Autodesk Inventor part; units mm, degrees
ref_plane "YZ Plane" through (0, 0, 0) normal (1, 0, 0) x (0, 1, 0)
ref_plane "XZ Plane" through (0, 0, 0) normal (0, 1, 0) x (-1, 0, 0)
ref_plane "XY Plane" through (0, 0, 0) normal (0, 0, 1) x (1, 0, 0)
sketch "Skizze2" plane through (0, 0, 0) normal (0, 1, 0) x (-1, 0, 0)
  line L0 (0, 0) -> (30, 0)
  line L1 (30, 0) -> (30, 30)
  line L2 (30, 30) -> (0, 30)
  line L3 (0, 30) -> (0, 0)
  line L4 (28, 28) -> (2, 28)
  line L5 (2, 28) -> (2, 2)
  line L6 (2, 2) -> (28, 2)
  line L7 (28, 2) -> (28, 28)
  line L8 (19, 30) -> (19, 28)
  line L9 (11, 30) -> (11, 28)
  line L10 (23.5, 28) -> (23.5, 25)
  line L11 (19.5, 21) -> (10.5, 21)
  line L12 (6.5, 25) -> (6.5, 28)
  line L13 (23.5, 25) -> (19.5, 21)
  line L14 (6.5, 25) -> (10.5, 21)
  line L15 (5, 6.5) -> (2, 6.5)
  line L16 (9, 19.5) -> (9, 10.5)
  line L17 (5, 23.5) -> (9, 19.5)
  line L18 (2, 23.5) -> (5, 23.5)
  line L19 (0, 19) -> (2, 19)
  line L20 (0, 11) -> (2, 11)
  line L21 (5, 6.5) -> (9, 10.5)
  line L22 (23.5, 5) -> (23.5, 2)
  line L23 (10.5, 9) -> (19.5, 9)
  line L24 (6.5, 5) -> (10.5, 9)
  line L25 (6.5, 2) -> (6.5, 5)
  line L26 (11, 0) -> (11, 2)
  line L27 (19, 0) -> (19, 2)
  line L28 (23.5, 5) -> (19.5, 9)
  line L29 (25, 23.5) -> (28, 23.5)
  line L30 (21, 10.5) -> (21, 19.5)
  line L31 (25, 6.5) -> (21, 10.5)
  line L32 (28, 6.5) -> (25, 6.5)
  line L33 (30, 11) -> (28, 11)
  line L34 (30, 19) -> (28, 19)
  line L35 (25, 23.5) -> (21, 19.5)
  circle A0 centre (15, 15) radius 3.5
  line L36 (20, 30) -> (20, 29)
  line L37 (20, 29) -> (19, 29)
  line L38 (11, 29) -> (10, 29)
  line L39 (10, 29) -> (10, 30)
  line L40 (1, 10) -> (0, 10)
  line L41 (1, 11) -> (1, 10)
  line L42 (1, 20) -> (1, 19)
  line L43 (0, 20) -> (1, 20)
  line L44 (20, 1) -> (20, 0)
  line L45 (19, 1) -> (20, 1)
  line L46 (10, 1) -> (11, 1)
  line L47 (10, 0) -> (10, 1)
  line L48 (29, 20) -> (30, 20)
  line L49 (29, 19) -> (29, 20)
  line L50 (29, 10) -> (29, 11)
  line L51 (30, 10) -> (29, 10)
  point P0 (23.5, 21)
  point P1 (6.5, 21)
  point P2 (9, 6.5)
  point P3 (9, 23.5)
  point P4 (23.5, 9)
  point P5 (6.5, 9)
  point P6 (21, 23.5)
  point P7 (21, 6.5)
  dimension "d23" = 30
  dimension "d24" = 30
  dimension "d25" = 2
  dimension "d26" = 2
  dimension "d27" = 2
  dimension "d28" = 2
  dimension "d29" = 8
  dimension "d30" = 11
  dimension "d32" = 6.5
  dimension "d33" = 17
  dimension "d34" = 9
  dimension "d35" = 4
  dimension "d36" = 4
  dimension "d37" = 4
  dimension "d38" = 4
  dimension "d39" = 15
  dimension "d40" = 15
  dimension "d43" = 360
  dimension "d45" = 7
  dimension "d46" = 1
  dimension "d47" = 1
  dimension "d48" = 1
  dimension "d49" = 1
  dimension "d52" = 360
extrude "Extrusion1" add sketch "Skizze2" along normal blind 123 contours L3 L40 L41 L20 L5 L6 L26 L46 L47 L0 | L44 L45 L27 L6 L7 L33 L50 L51 L1 L0 | L3 L2 L39 L38 L9 L4 L5 L19 L42 L43 | L6 L5 L15 L21 L16 L17 L18 L4 L12 L14 L11 L13 L10 L7 L29 L35 L30 L31 L32 L22 L28 L23 L24 L25 | L48 L49 L34 L7 L4 L8 L37 L36 L2 L1
fillet "Rundung1" radius 2 4 edges at (0, 61.5, 30) (0, 61.5, 0) (-30, 61.5, 0) (-30, 61.5, 30)
properties part number "ITEM_Profil"
Can you work these out from the model? Positions are in its coordinate system, mm. A direction names the side the tool comes from. Coordinates: 2 decimals unless noted, no trailing zeros. Order: outer loops, then holes, each group sorted by start corner. A loop starts at its lowest first (then second) coordinate and runs counter-clockwise, first axis right, second up. Notation, with made-up numbers: M 68,-16.75 L 127,-16.75 A22 ccw 127,-9.75 Z; hole C 19,-20 d5. An arc over 180 degrees is marked long. Write item = value, one per line.
(1) Suppose I cut it at B-B on z = 15. Please give me the cut outline in (x, y).
Results are:
outline = M -21,0 L -18.5,0 L -18.5,123 L -21,123 Z; M -11.5,0 L -9,0 L -9,123 L -11.5,123 Z
(2) If we mould it in two halves opening along X, with no side actions, what happens to faces 3 (the face through (-24, 61, 0)), 4 (the face through (-30, 61, 24)), 5 (the face through (-6.5, 61, 3))? For each: pulls with the +X half, pulls with the -X half, needs draft (parallel to the pull), parting line crosses it, or undercut.
Results are:
face_3 = needs draft
face_4 = pulls with the -X half
face_5 = undercut
(3) For faces 1 (the face through (-0.57, 62.36, 0.6)), 2 (the face through (-23.5, 61, 27)), which set-ups out of +Z, -Z, +X, -X, +Y, -Y let a thin tool reach every point of the face, with its end or its side?
Results are:
face_1 = -Z, +X, +Y, -Y
face_2 = +Y, -Y
(4) Suppose I cut it at A-A on x = -15. Please give me the cut outline in (y, z), plus the area to 3 significant figures.
Results are:
outline = M 0,9 L 123,9 L 123,11.5 L 0,11.5 Z; M 0,18.5 L 123,18.5 L 123,21 L 0,21 Z
area = 615 mm2
(5) I need wall thicknesses on line 1 along X through (y, z) = (117.5, 19.25); line 2 along Z through (x, y) = (-15, 53.5); line 3 along X through (y, z) = (48.5, 25.5). Which ranges of each line are inside material? Lowest first, please. Write a range as [from, to].
Results are:
line_1 = [-29, -28], [-21, -9], [-2, -1]
line_2 = [9, 11.5], [18.5, 21]
line_3 = [-30, -23.5], [-6.5, 0]
(6) For pin 1 Ø2.5 at (y, z) = (77.5, 13.5) entering from -X; pin 2 Ø4.5 at (y, z) = (88.5, 15.5) entering from +X; pin 3 Ø1.5 at (y, z) = (103.5, 11.5) entering from +X, each with a flat end and sliding along its axis, tell me the tip position at first contact or that it passes through.
Results are:
pin_1 = -21
pin_2 = -9
pin_3 = -1
